Autodesk Inventor part; units mm, degrees
ref_plane "YZ Plane" through (0, 0, 0) normal (1, 0, 0) x (0, 1, 0)
ref_plane "XZ Plane" through (0, 0, 0) normal (0, 1, 0) x (-1, 0, 0)
ref_plane "XY Plane" through (0, 0, 0) normal (0, 0, 1) x (1, 0, 0)
sketch "Sketch1" plane through (0, 0, 0) normal (0, 0, 1) x (1, 0, 0)
  line L0 (0, 0) -> (0, 22.958) construction
  line L1 (0, 0) -> (0, -22.958) construction
  line L2 (0, -22.958) -> (16.63, -22.958) construction
  line L3 (16.63, -22.958) -> (16.63, -81.958) construction
  line L4 (16.63, -81.958) -> (0, -81.958) construction
  line L5 (0, -81.958) -> (0, -22.958) construction
  line L6 (0, 22.958) -> (16.63, 22.958) construction
  line L7 (16.63, 22.958) -> (16.63, 81.958) construction
  line L8 (16.63, 81.958) -> (0, 81.958) construction
  line L9 (0, 81.958) -> (0, 22.958) construction
  line L10 (0, -52.458) -> (0.5, -52.458) construction
  line L11 (8.315, -22.958) -> (8.315, -23.458) construction
  line L12 (0, 0) -> (-53.686, 0) construction
  circle A0 centre (-53.686, 0) radius 74 construction
  line L13 (20.314, 0) -> (20.814, 0) construction
  line L14 (16.63, -22.958) -> (17.13, -22.958) construction
  line L15 (16.63, 22.958) -> (17.13, 22.958) construction
  line L16 (0.5, -23.458) -> (17.13, -23.458)
  line L17 (17.13, -23.458) -> (17.13, -81.958)
  line L18 (17.13, -81.958) -> (0.5, -81.958)
  line L19 (0.5, -81.958) -> (0.5, -23.458)
  line L20 (8.315, 22.958) -> (8.315, 23.458) construction
  line L21 (0.5, 81.958) -> (17.13, 81.958)
  line L22 (17.13, 81.958) -> (17.13, 23.458)
  line L23 (17.13, 23.458) -> (0.5, 23.458)
  line L24 (0.5, 23.458) -> (0.5, 81.958)
  arc A1 (17.13, -23.458) -> (17.13, 23.458) centre (-55.7128, 0) ccw
  line L25 (17.13, -81.958) -> (23.13, -81.958)
  line L26 (23.13, -81.958) -> (23.13, 81.958)
  line L27 (23.13, 81.958) -> (17.13, 81.958)
  dimension "d8" = 148
  dimension "d0" = 22.958
  dimension "d1" = 22.958
  dimension "d2" = 16.63
  dimension "d3" = 59
  dimension "d5" = 0.5
  dimension "d6" = 0.5
  dimension "d7" = 53.686
  dimension "d9" = 0.5
  dimension "d10" = 0.5
  dimension "d11" = 0.5
  dimension "d13" = 0.5
  dimension "d14" = 6
extrude "Extrusion1" add sketch "Sketch1" along normal blind 9
sketch "Sketch2" plane through (0, 0, 0) normal (0, 0, -1) x (-1, 0, 0)
  line L0 (-16.63, 22.958) -> (-16.63, 81.958) construction
  circle A0 centre (53.686, 0) radius 74 construction
  line L1 (-16.63, -22.958) -> (-16.63, -81.958) construction
  line L2 (-0.5, 23.458) -> (-17.13, 23.458)
  line L3 (-16.63, 23.458) -> (-16.63, 81.958)
  line L4 (-23.13, 81.958) -> (-0.5, 81.958)
  line L5 (-17.13, -23.458) -> (-0.5, -23.458)
  line L6 (-16.63, -23.458) -> (-16.63, -81.958)
  line L7 (-0.5, -81.958) -> (-23.13, -81.958)
  arc A1 (-17.13, 23.458) -> (-17.13, -23.458) centre (55.7128, 0) ccw
  arc A2 (-17.13, 23.458) -> (-17.13, -23.458) centre (55.7128, 0) ccw
  line L8 (-23.13, 81.958) -> (-110.13, 81.958)
  line L9 (-110.13, 81.958) -> (-110.13, -81.958)
  line L10 (-110.13, -81.958) -> (-23.13, -81.958)
  line L11 (-23.13, -81.958) -> (-23.13, 81.958)
  line L12 (0, 0) -> (-10.5, 0) construction
  line L13 (-0.5, -81.958) -> (-23.13, -81.958)
  arc A3 (-10.5, 38.3695) -> (-10.5, -38.3695) centre (55.7128, 0) ccw
  line L14 (-10.5, 38.3695) -> (-10.5, 81.958)
  line L15 (-10.5, -38.3695) -> (-10.5, -81.958)
  point P0 (-10, 81.958)
  dimension "d17" = 87
  dimension "d66" = 10.5
extrude "Extrusion2" add sketch "Sketch2" along normal blind 7 and the other way blind 2 contours A1 A3 L6 L7 L11 L4 L3 | L3 L4 L14 A3 | A3 L15 L7 L6 | L11 L10 L9 L8
sketch "Sketch3" plane through (0, 0, 9) normal (0, 0, 1) x (1, 0, 0)
  line L0 (0.5, -81.958) -> (23.13, -81.958) construction
  line L1 (0, -23.458) -> (10, -23.458) construction
  line L2 (10, -23.458) -> (10, -81.958) construction
  line L3 (10, -81.958) -> (0, -81.958) construction
  line L4 (0, -81.958) -> (0, -23.458) construction
  line L5 (0, 23.458) -> (10, 23.458) construction
  line L6 (0, 81.958) -> (0, 23.458) construction
  line L7 (5, -81.958) -> (5, -71.958) construction
  line L8 (17.13, -23.458) -> (0.5, -23.458) construction
  line L9 (5, -23.458) -> (5, -33.458) construction
  line L10 (5, -23.458) -> (15, -23.458) construction
  circle A0 centre (5, -71.958) radius 1.75
  circle A1 centre (5, -33.458) radius 1.75
  line L11 (-21.548, 0) -> (41.2165, 0) construction
  circle A2 centre (5, 71.958) radius 1.75
  circle A3 centre (5, 33.458) radius 1.75
  point P0 (0, 0)
  dimension "d20" = 10
  dimension "d21" = 10
  dimension "d22" = 10
  dimension "d24" = 3.5
  dimension "d25" = 3.5
extrude "Extrusion3" cut sketch "Sketch3" against normal up to surface (9 mm away)
sketch "Sketch4" plane through (0, 0, 9) normal (0, 0, 1) x (1, 0, 0)
  circle A0 centre (5, -71.958) radius 1.75
  circle A1 centre (5, -71.958) radius 2.65
  circle A2 centre (5, -33.458) radius 1.75
  circle A3 centre (5, -33.458) radius 2.65
  circle A4 centre (5, 33.458) radius 1.75
  circle A5 centre (5, 33.458) radius 2.65
  circle A6 centre (5, 71.958) radius 1.75
  circle A7 centre (5, 71.958) radius 2.65
  point P0 (0, 0)
  dimension "d28" = 5.3
  dimension "d29" = 5.3
extrude "Extrusion4" cut sketch "Sketch4" against normal blind 6 contours A0 | A1 | A2 | A3 | A4 | A5 | A6 | A7
sketch "Sketch5" plane through (0, 0, 2) normal (0, 0, 1) x (1, 0, 0)
  line L0 (23.13, -71.958) -> (105.13, -71.958)
  line L1 (105.13, -71.958) -> (105.13, 32.042)
  line L2 (105.13, 32.042) -> (23.13, 32.042)
  line L3 (23.13, 32.042) -> (23.13, -71.958)
  line L4 (31.2383, 46.3792) -> (79.2383, 46.3792)
  line L5 (79.2383, 46.3792) -> (79.2383, 71.3792)
  line L6 (79.2383, 71.3792) -> (31.2383, 71.3792)
  line L7 (31.2383, 71.3792) -> (31.2383, 46.3792)
  line L8 (23.13, -81.958) -> (23.13, 81.958) construction
  line L9 (23.13, -81.958) -> (23.13, 81.958) construction
  line L10 (23.13, -81.958) -> (23.13, -71.958) construction
  point P0 (0, 0)
  dimension "d34" = 82
  dimension "d35" = 104
  dimension "d36" = 48
  dimension "d37" = 25
  dimension "d38" = 10
extrude "Extrusion5" cut sketch "Sketch5" against normal blind 3.5
sketch "Sketch6" plane through (0, 0, 2) normal (0, 0, 1) x (1, 0, 0)
  line L0 (23.13, 32.042) -> (105.13, 32.042)
  line L1 (64.13, 32.042) -> (39.13, 32.042)
  line L2 (64.13, 32.042) -> (89.13, 32.042)
  line L3 (89.13, 32.042) -> (89.13, 25.042)
  line L4 (89.13, 25.042) -> (39.13, 25.042)
  line L5 (39.13, 25.042) -> (39.13, 32.042)
  point P0 (0, 0)
  dimension "d41" = 25
  dimension "d42" = 25
  dimension "d43" = 7
extrude "Extrusion6" cut sketch "Sketch6" against normal up to surface (9 mm away)
sketch "Sketch7" plane through (23.13, 32.042, 2) normal (0, -1, 0) x (1, 0, 0)
  line L0 (66, -9) -> (16, -9)
  line L1 (66, -3.5) -> (66, -9)
  line L2 (16, -9) -> (66, -9)
  line L3 (66, -9) -> (66, -6)
  line L4 (66, -6) -> (16, -6)
  line L5 (16, -6) -> (16, -9)
  point P0 (-23.13, -2)
  dimension "d46" = 3
extrude "Extrusion7" cut sketch "Sketch7" against normal up to surface (49.916 mm away)
sketch "Sketch8" plane through (0, 0, -1.5) normal (0, 0, 1) x (1, 0, 0)
  line L0 (41.13, -49.8888) -> (87.13, -49.8888)
  line L1 (87.13, -49.8888) -> (87.13, -3.8888)
  line L2 (87.13, -3.8888) -> (41.13, -3.8888)
  line L3 (41.13, -3.8888) -> (41.13, -49.8888)
  line L4 (41.13, -49.8888) -> (87.13, -3.8888) construction
  line L5 (87.13, -49.8888) -> (41.13, -3.8888) construction
  point P0 (0, 0)
  point P1 (64.13, -26.8888)
  dimension "d49" = 46
  dimension "d50" = 46
extrude "Extrusion8" cut sketch "Sketch8" against normal up to surface (5.5 mm away)
sketch "Sketch9" plane through (0, 0, 2) normal (0, 0, 1) x (1, 0, 0)
  line L0 (110.13, 81.958) -> (110.13, -81.958)
  line L1 (110.13, -81.958) -> (120.13, -81.958)
  line L2 (120.13, -81.958) -> (120.13, 81.958)
  line L3 (120.13, 81.958) -> (110.13, 81.958)
  line L4 (110.13, 81.958) -> (110.13, -81.958)
  point P0 (0, 0)
  dimension "d53" = 10
extrude "Extrusion9" add sketch "Sketch9" against normal blind 9
sketch "Sketch10" plane through (0, 0, 2) normal (0, 0, 1) x (1, 0, 0)
  line L0 (105.13, 32.042) -> (105.13, -71.958) construction
  line L1 (105.13, -71.958) -> (120.13, -71.958) construction
  line L2 (120.13, -81.958) -> (120.13, 81.958) construction
  circle A0 centre (112.63, -67.7077) radius 1.275
  circle A1 centre (112.63, 66.21) radius 1.275
  circle A2 centre (112.63, 20.0315) radius 1.275
  line L3 (23.13, -81.958) -> (120.13, -81.958) construction
  line L4 (112.63, 66.21) -> (112.63, 81.958) construction
  line L5 (89.13, 81.958) -> (120.13, 81.958) construction
  line L6 (112.63, 66.21) -> (112.63, 20.0315) construction
  line L7 (112.63, -67.7077) -> (112.63, -81.958) construction
  point P0 (0, 0)
  dimension "d56" = 2.55
  dimension "d57" = 2.55
  dimension "d58" = 2.55
  dimension "d60" = 15.748
  dimension "d61" = 46.1785
  dimension "d62" = 14.2503
extrude "Extrusion10" cut sketch "Sketch10" against normal blind 4.5
fillet "Fillet1" radius 6 6 edges at (41.13, -49.8888, -4.25) (41.13, -3.8888, -4.25) (87.13, -3.8888, -4.25) (87.13, -49.8888, -4.25) (23.13, 81.958, 5.5) (23.13, -81.958, 5.5)
properties part number "Base Extension 1"
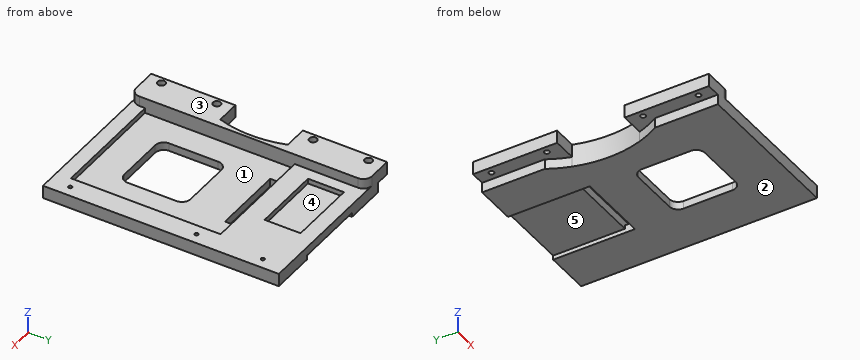
The listing builds one solid part. Answer for the finished solid, in the listing's coordinates (mm). Face numbers are marked on the shaded views. A direction names the side the tool comes from. Round coordinates to 2 decimals unless told otherwise and drop trailing zeros. Loops run counter-clockwise (first coordinate to the right, second up) from the corner with the lowest first, then second, coordinate; pieces in that order, holes last. Notation, with made-up numbers: M -3,67.25 L 45,67.25 A19 cw 45,84.25 Z; hole C 44.25,-18.5 d3. An arc over 180 degrees is marked long. Write each question's results on one line, items separated by ' | '. Start each with the question number.
1) Each of these flat-tipped pins is pushed along its axis until it touches: pin 1 (1 mm diameter, centred on y = 63, z = -5, fed in from -X); pin 2 (12 mm diameter, centred on x = 62, y = -61, fed in from +Z); pin 3 (1.6 mm diameter, centred on x = 5, y = 33.5, fed in from +Z); pin 4 (8 mm diameter, centred on x = 99.5, y = 47.5, fed in from +Z). Where does it stop, or does it pass through?
2) Straight lines are drawn through the part: probe 1 along Y at (x, z) = (5, 1.15); probe 2 along Y at (x, z) = (112.63, 0.15) (1 decimal); probe 3 along Y at (x, z) = (5, 6). For each, find the intervals that lie inside material, in ascending order.
3) Find section C-C on x = 33.5. Write down the section's boundary in (y, z).
4) Determine the mould class of the marked faces 1 and 2 for opening direction Y: pulls with the +Y half, pulls with the -Y half, needs draft (parallel to the pull), parting line crosses it, or undercut.
5) Find section B-B on y = 27.5. Write down the section's boundary in (x, z).
6) Find section A-A on x = 69.5. Write down the section's boundary in (y, z).
7) Find section D-D on z = 6.75. Write down the section's boundary in (x, y), plus the area to 3 significant figures.
8) Which of the six approach directions +Z, -Z, +X, -X, +Y, -Y give full straight-line access (tool end or side, diameter ignored) to the marked faces 3, 4 and 5?
Final values:
1) pin 1: x = 10.5 | pin 2: z = -1.5 | pin 3: through | pin 4: z = 2
2) probe 1: -81.96 to -73.71, -70.21 to -35.21, -31.71 to -23.46, 23.46 to 31.71, 35.21 to 70.21, 73.71 to 81.96 | probe 2: -82 to -69, -66.4 to 18.8, 21.3 to 64.9, 67.5 to 82 | probe 3: -81.96 to -74.61, -69.31 to -36.11, -30.81 to -23.46, 23.46 to 30.81, 36.11 to 69.31, 74.61 to 81.96
3) outline: M -81.96,-7 L 81.96,-7 L 81.96,2 L 71.38,2 L 71.38,-1.5 L 46.38,-1.5 L 46.38,2 L 32.04,2 L 32.04,-1.5 L -71.96,-1.5 L -71.96,2 L -81.96,2 Z
4) face 1: undercut | face 2: needs draft
5) outline: M 0.5,0 L 15.7,0 L 15.7,-7 L 39.13,-7 L 39.13,-1.5 L 23.13,-1.5 L 23.13,9 L 0.5,9 Z; M 89.13,-7 L 120.13,-7 L 120.13,2 L 105.13,2 L 105.13,-1.5 L 89.13,-1.5 Z
6) outline: M -81.96,-7 L -49.89,-7 L -49.89,-1.5 L -71.96,-1.5 L -71.96,2 L -81.96,2 Z; M -3.89,-7 L 25.04,-7 L 25.04,-1.5 L -3.89,-1.5 Z; M 32.04,-4 L 81.96,-4 L 81.96,2 L 71.38,2 L 71.38,-1.5 L 46.38,-1.5 L 46.38,2 L 32.04,2 Z
7) outline: M 0.5,-81.96 L 17.13,-81.96 A6 ccw 23.13,-75.96 L 23.13,75.96 A6 ccw 17.13,81.96 L 0.5,81.96 L 0.5,23.46 L 17.13,23.46 A76.53 cw 17.13,-23.46 L 0.5,-23.46 Z; hole C 5,-71.96 d5.3; hole C 5,-33.46 d5.3; hole C 5,33.46 d5.3; hole C 5,71.96 d5.3 | area: 2,710 mm²
8) face 3: +Z, +X, -X, +Y, -Y | face 4: +Z | face 5: -Z, +Y
